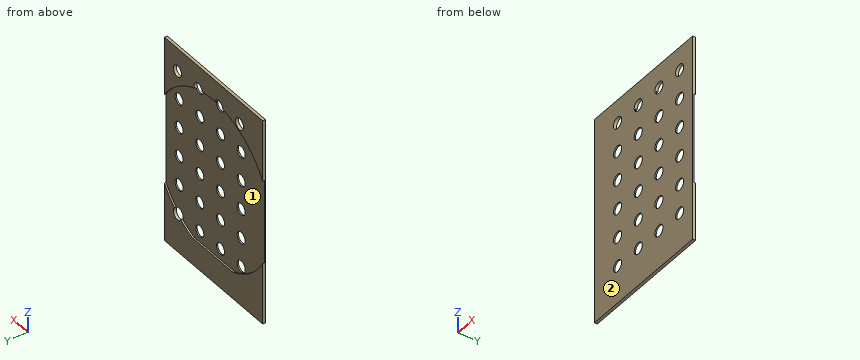
Autodesk Inventor part; units mm, degrees
ref_plane "YZ Plane" through (0, 0, 0) normal (1, 0, 0) x (0, 1, 0)
ref_plane "XZ Plane" through (0, 0, 0) normal (0, 1, 0) x (-1, 0, 0)
ref_plane "XY Plane" through (0, 0, 0) normal (0, 0, 1) x (1, 0, 0)
sketch "Sketch1" plane through (0, 0, 0) normal (0, 1, 0) x (-1, 0, 0)
  line L0 (0, 0) -> (85.48, 0)
  line L1 (85.48, 0) -> (85.48, -127.76)
  line L2 (85.48, -127.76) -> (0, -127.76)
  line L3 (0, -127.76) -> (0, 0)
  line L4 (42.74, -127.76) -> (42.74, -63.879)
  circle A0 centre (42.1561, -63.879) radius 50.5
  line L5 (26.485, -111.163) -> (58.985, -111.1664)
  line L6 (42.74, -63.879) -> (42.7347, -113.879)
  line L7 (26.485, -111.163) -> (24.4227, -111.163)
  line L8 (58.985, -111.1664) -> (59.8896, -111.163)
  point P0 (85.48, -37.9311)
  point P1 (85.48, -89.8269)
  point P2 (0, -91.6839)
  point P3 (0, -36.0741)
  point P4 (42.735, -111.1647)
  point P5 (42.74, -111.1647)
  point P6 (42.74, -114.3756)
  dimension "d0" = 85.48
  dimension "d1" = 127.76
  dimension "d2" = 63.881
  dimension "d3" = 101
  dimension "d4" = 32.5
extrude "Extrusion1" add sketch "Sketch1" along normal blind 1.7938 contours L0 L1 A0 L3 | A0 L4 L2 L3 | L1 L2 L4 A0 | L7 L5 L4 A0 | A0 L4 L5 L8
extrude "Extrusion2" add sketch "Sketch1" along normal blind 0.7937 contours A0 L1 L8 L5 L4 L6 L7 L3 | L7 L5 L4 A0 | A0 L4 L5 L8 | L5 L6 L4
sketch "Sketch2" plane through (0, 1.7938, 0) normal (0, 1, 0) x (1, 0, 0)
  line L0 (-85.48, 127.76) -> (-85.48, 0)
  line L1 (-85.48, 25.2748) -> (-79.48, 25.2748)
  line L2 (-85.48, 25.2748) -> (-79.48, 25.2748) construction
  arc A0 (-85.48, 37.9311) -> (0, 36.0741) centre (-42.1561, 63.879) ccw
  line L3 (-42.1561, 13.379) -> (-42.1561, 19.379)
  line L4 (-42.1561, 19.379) -> (-85.48, 19.379)
  line L5 (-85.48, 19.379) -> (-79.48, 19.379)
  line L6 (0, 0) -> (0, 14.38)
  line L7 (0, 0) -> (0, 127.76)
  line L8 (0, 14.38) -> (-11.34, 14.38)
  dimension "d9" = 6
  dimension "d10" = 0
  dimension "d24" = 6
  dimension "d25" = 6
  dimension "d26" = 14.38
  dimension "d27" = 11.34
hole "Hole1" at (-11.34, 1.7938, -14.38) direction (0, -1, 0) diameter 7 end through all
pattern_linear "Rectangular Pattern1" count 6 spacing 18 along (0, 0, -1) count 4 spacing 18 along (-1, 0, 0) of "Hole1"
properties part number "100mm wafer wellplate - corral mask - with flat - lowdensity"
Model file for the job. Use its own axes, mm. Face numbers are marked on the shaded views. Round coordinates to 2 decimals unless told otherwise and drop trailing zeros. Write each loop counter-clockwise with the first axis right and the second up, starting at its lowest first coordinate (ties: lowest second). Pieces come first, ordered by that corner, then holes. Notation, with made-up numbers: M 45.5,8 L 70.5,8 A7 ccw 70.5,13 Z; hole C -33,81.5 d2. An arc over 180 degrees is marked long. Put each result on its own line as item: value.
Item 1: Cut at D-D (x = -72.5). List the corners of the cut face in (y, z).
Responses:
outline: M 0,-127.76 L 1.79,-127.76 L 1.79,-104.25 L 0.79,-104.25 L 0.79,-23.51 L 1.79,-23.51 L 1.79,0 L 0,0 Z
Item 2: Cut at C-C (y = 1.25). List the corners of the cut face in (x, z) (3 decimals), and give its area (3 significant figures).
Responses:
outline: M -85.48,-127.76 L 0,-127.76 L 0,-91.684 A50.5 cw -8.894,-101.877 A3.5 cw long -14.405,-106.07 A50.5 cw -24.423,-111.163 L -26.485,-111.163 L -58.985,-111.166 L -59.89,-111.163 A50.5 cw -85.48,-89.827 Z; M -85.48,-37.931 A50.5 cw -50.831,-14.13 A3.5 cw -43.977,-13.412 A50.5 cw -32.837,-14.246 A3.5 cw long -26.217,-15.96 A50.5 cw 0,-36.074 L 0,0 L -85.48,0 Z; hole C -65.34,-14.38 d7; hole C -11.34,-14.38 d7
area: 3,410 mm²
Item 3: Cut at B-B (x = -29.34). State how many separate pieces and enclosed holes the cut face has, and give its area (3 significant figures).
Responses:
separate pieces: 7
enclosed holes: 0
area: 95.5 mm²
Item 4: Cut at A-A (z = -50.38). List the corners of the cut face in (x, y), and give its area (3 significant figures).
Responses:
outline: M -85.48,0 L -68.84,0 L -68.84,0.79 L -85.48,0.79 Z; M -61.84,0 L -50.84,0 L -50.84,0.79 L -61.84,0.79 Z; M -43.84,0 L -32.84,0 L -32.84,0.79 L -43.84,0.79 Z; M -25.84,0 L -14.84,0 L -14.84,0.79 L -25.84,0.79 Z; M -7.84,0 L 0,0 L 0,0.79 L -7.84,0.79 Z
area: 45.6 mm²
Item 5: Mould opens along X. For the marked faces 1 and 2 say: +X half, -X half, draft (parallel to the pull), parting line (faces both ways), or undercut.
Responses:
face 1: undercut
face 2: draft
Item 6: Probe L1, parallel to X at y = 0.3, z = -32.38; L2, parallel to Y at x = -27, z = -58.5; L3, parallel to Z at x = -50.5, y = 1.45. List the from-to ranges inside material, lowest first. Write a range as from..to.
Responses:
L1: -85.48..-68.84, -61.84..-50.84, -43.84..-32.84, -25.84..-14.84, -7.84..0
L2: 0..0.79
L3: -127.76..-111.17, -12.88..0
Item 7: Flat gauge pins, fed straight in: P1, Ø12, axis at x = -9, z = -57, coming from the +Y side; P2, Ø5.5, axis at x = -65.34, z = -86.38, coming from the +Y side. Where does each tip first touch, or does it go through?
Responses:
P1: y = 0.79
P2: through
